from build123d import *

# Parameters (mm, degrees)
F0_W     = 3.175
F0_H     = 10.16
F1_DEPTH = 3.175


with BuildPart() as f1:
    # F0 (on Top) → F1 (new body)
    with BuildSketch(Plane.XY):
        Polygon((-138.043921, -60.22932), (-138.043921, -64.061883), (-72.003921, -64.061883), (-72.003921, -8.181883), (-77.367083, -8.181883), (-84.703921, -8.181883), (-84.703921, -11.356883), (-97.403921, -11.356883), (-97.403921, -8.181883), (-122.803921, -8.181883), (-122.803921, 25.984842), (-125.978921, 25.984842), (-125.978921, 38.684842), (-122.803921, 38.684842), (-122.803921, 64.084842), (-125.978921, 64.084842), (-125.978921, 76.784842), (-122.803921, 76.784842), (-122.803921, 93.418117), (-138.043921, 93.418117), (-138.043921, 21.05068), (-131.693921, 21.05068), (-131.693921, -60.22932), align=None)
        with Locations((-104.071421, -48.821883)):
            Rectangle(F0_W, F0_H, mode=Mode.SUBTRACT)
        with Locations((-104.071421, -23.421883)):
            Rectangle(F0_W, F0_H, mode=Mode.SUBTRACT)
        Polygon((-72.003921, -8.181883), (-72.003921, -64.061883), (-5.963921, -64.061883), (-5.963921, -60.22932), (-12.313921, -60.22932), (-12.313921, 21.05068), (-5.963921, 21.05068), (-5.963921, 93.418125), (-21.203921, 93.418125), (-21.203921, 76.784842), (-18.028921, 76.784842), (-18.028921, 64.084842), (-21.203921, 64.084842), (-21.203921, 38.684842), (-18.028921, 38.684842), (-18.028921, 25.984842), (-21.203921, 25.984842), (-21.203921, -8.181883), (-26.567083, -8.181883), (-46.603921, -8.181883), (-46.603921, -11.356883), (-59.303921, -11.356883), (-59.303921, -8.181883), align=None)
        with Locations((-39.936421, -48.821883)):
            Rectangle(F0_W, F0_H, mode=Mode.SUBTRACT)
        with Locations((-39.936421, -23.421883)):
            Rectangle(F0_W, F0_H, mode=Mode.SUBTRACT)
    extrude(amount=F1_DEPTH)


solid = f1.part
Could you check a few things on this model? Use its own coordinates, in mm. A direction names the side the tool comes from. Round coordinates to 2 decimals unless told otherwise and drop trailing zeros. Loops run counter-clockwise (first coordinate to the right, second up) from the corner with the lowest first, then second, coordinate; pieces in that order, holes last. Notation, with made-up numbers: (-33, -39) - (-23, -39) arc R9 ccw to (-23, -35) - close; hole circle Ø6 at (53.25, 59). An arc over 180 degrees is marked (long way). Write item = value, one per line.
1) I need wall thicknesses on line 1 along Y through (x, z) = (-40.5, 2); line 2 along X through (y, z) = (-45.5, 1.85); line 3 along X through (y, z) = (28, 0.55). Which ranges of each line are inside material? Lowest first, please. Write a range as from..to.
Computed:
line_1 = -64.06..-53.9, -43.74..-28.5, -18.34..-8.18
line_2 = -131.69..-105.66, -102.48..-41.52, -38.35..-12.31
line_3 = -138.04..-125.98, -18.03..-5.96
2) Imagine slicing it at A-A (y = 40.5). Please give me the cut outline in (x, z) (3 decimals), and give its area (3 significant figures).
Computed:
outline = (-138.044, 0) - (-122.804, 0) - (-122.804, 3.175) - (-138.044, 3.175) - close; (-21.204, 0) - (-5.964, 0) - (-5.964, 3.175) - (-21.204, 3.175) - close
area = 96.8 mm2
3) Imagine slicing it at D-D (x = -95). Please give me the cut outline in (y, z) (3 decimals), and give its area (3 significant figures).
Computed:
outline = (-64.062, 0) - (-11.357, 0) - (-11.357, 3.175) - (-64.062, 3.175) - close
area = 167 mm2
4) Imagine slicing it at B-B (y = -1.5). Please give me the cut outline in (x, z) (3 decimals).
Computed:
outline = (-131.694, 0) - (-122.804, 0) - (-122.804, 3.175) - (-131.694, 3.175) - close; (-21.204, 0) - (-12.314, 0) - (-12.314, 3.175) - (-21.204, 3.175) - close
5) If we mould it in two halves opening along X, with no side actions, what happens to faces 1 (the flat face through (-105.659, -23, 2)), 2 (the flat face through (-5.964, -62, 2)), 3 (the flat face through (-13, 93.418, 2))? For each: pulls with the +X half, pulls with the -X half, needs draft (parallel to the pull), parting line crosses it, or undercut.
Computed:
face_1 = undercut
face_2 = pulls with the +X half
face_3 = needs draft
6) I'm going to push flat-ended pins straight in: P1, Ø1, axis at y = -9.5, z = 2, coming from the +X side; P2, Ø3, axis at x = -43.5, y = -25.5, coming from the -Z side; P3, Ø1.6, axis at x = -71.5, z = 1.5, coming from the +Y side; P4, Ø1, axis at x = -94, z = 1, coming from the +Y side. Where does each tip first touch, or does it pass through?
Computed:
P1 = -12.31
P2 = 0
P3 = -8.18
P4 = -11.36
7) Imagine slicing it at C-C (z = 0.5). Give the number of separate pieces and of enclosed holes in the cut face, and give its area (3 significant figures).
Computed:
separate_pieces = 1
enclosed_holes = 4
area = 9,070 mm2
8) On a 3-axis mill with a long thin cutter (end or side, diameter ignored), from which of +Z, -Z, +X, -X, +Y, -Y can I reach the whole of each face in a straight line? I mean faces 4 (the flat face through (-40, -28.502, 2)), 5 (the flat face through (-73, -19, 3.175)), 6 (the flat face through (-21.204, 52, 2)), 7 (the flat face through (-135, -60.229, 2)). Say none if no direction works.
Computed:
face_4 = +Z, -Z
face_5 = +Z, +X, -X, +Y, -Y
face_6 = +Z, -Z, +Y
face_7 = +Z, -Z, -X
